Autodesk Inventor part; units mm, degrees
ref_plane "Start Plane" through (0, 0, -13.5858) normal (0, 0, 1) x (1, 0, 0)
ref_plane "End Plane" through (0, 0, 2013.5858) normal (0, 0, 1) x (1, 0, 0)
ref_plane "Work Plane4" through (0, -15.7071, 2014.2929) normal (0, 0.7071, 0.7071) x (1, 0, 0)
ref_plane "Start Plane" through (0, 0, -13.5858) normal (0, 0, 1) x (1, 0, 0)
ref_plane "End Plane" through (0, 0, 2013.5858) normal (0, 0, 1) x (1, 0, 0)
sketch "Sketch" plane through (0, 0, 0) normal (0, 0, 1) x (1, 0, 0)
  line L0 (-15, -12) -> (-15, 12)
  line L1 (-12, 15) -> (12, 15)
  line L2 (15, 12) -> (15, -12)
  line L3 (12, -15) -> (-12, -15)
  arc A0 (-15, -12) -> (-12, -15) centre (-12, -12) ccw
  arc A1 (-12, 15) -> (-15, 12) centre (-12, 12) ccw
  arc A2 (15, 12) -> (12, 15) centre (12, 12) ccw
  arc A3 (12, -15) -> (15, -12) centre (12, -12) ccw
  arc A4 (-12, 13) -> (-13, 12) centre (-12, 12) ccw
  line L4 (-12, 13) -> (12, 13)
  arc A5 (13, 12) -> (12, 13) centre (12, 12) ccw
  line L5 (13, 12) -> (13, -12)
  arc A6 (12, -13) -> (13, -12) centre (12, -12) ccw
  line L6 (12, -13) -> (-12, -13)
  arc A7 (-13, -12) -> (-12, -13) centre (-12, -12) ccw
  line L7 (-13, -12) -> (-13, 12)
  line L8 (0, 21.8698) -> (0, -21.8698) construction
  line L9 (-21.8698, 0) -> (21.8698, 0) construction
  dimension "d7" = 3
  dimension "d10" = 30
  dimension "d11" = 30
  dimension "d12" = 2
  dimension "d15" = 15
  dimension "d16" = 15
extrude "Body" add sketch "Sketch" along normal up to surface (2027.1716 mm away) from surface at -13.5858
sketch "Sketch3" plane through (0, 0, 0) normal (0, 0, 1) x (1, 0, 0)
  line L0 (0, 0) -> (10, 0)
ref_plane "Work Plane3" through (0, 0, 0) normal (0, -1, 0) x (1, 0, 0)
ref_plane "Work Plane4" through (0, -15.7071, 2014.2929) normal (0, 0.7071, 0.7071) x (1, 0, 0)
split "Split1" plane through (0, -15.7071, 2014.2929) removes the side toward (0, 0.7071, 0.7071)
ref_plane "Work Plane5" through (0, -15.7071, -14.2929) normal (0, 0.7071, -0.7071) x (1, 0, 0)
split "Split2" plane through (0, -15.7071, -14.2929) removes the side toward (0, 0.7071, -0.7071)
sketch "Sketch4" plane through (0, 0, 0) normal (0, -1, 0) x (1, 0, 0)
  line L0 (-2, -13.5858) -> (12, -13.5858)
  line L1 (-2, 2013.5858) -> (12, 2013.5858)
  dimension "d18" = 2027.1716
equation "\"d7\" = G_IR"
equation "\"d10\" = G_H"
equation "\"d11\" = G_W"
equation "\"d12\" = G_T"
equation "\"d15\" = 0.5 * d10"
equation "\"d16\" = 0.5 * d11"
equation "\"d3\" = G_L"
equation "\"G_W\" = 30"
equation "\"G_H\" = 30"
equation "\"G_T\" = 2"
equation "\"G_IR\" = 3"
equation "\"G_L\" = d18"
equation "\"G_OFFSET_START\" = 13.58579"
equation "\"G_OFFSET_END\" = 13.58579"
equation "\"d13\" = -G_OFFSET_START"
equation "\"d14\" = G_OFFSET_END + B_L"
properties part number "ISO 12633-2 - 30x30x2 - 2027,17" material "Steel, Mild"
Here's how the part is built. I have some questions about the finished solid (model axes, mm). Coordinates: 2 decimals unless noted, no trailing zeros. Loops run counter-clockwise (first coordinate to the right, second up) from the corner with the lowest first, then second, coordinate; pieces in that order, holes last. Notation, with made-up numbers: (-28.75, -39) -> (-13.75, -39) arc R18 cw to (-13.75, -20) -> close; hole circle Ø3 at (44.5, 77). An arc over 180 degrees is marked (long way). Use one line per item in the form item = value. Start each with the question number.
(1) Will this pin go through, and if not, where does the flat tip stop? pin 1 (10 mm diameter, centred on x = 9, y = -5.5, fed in from -Z).
(2) If we section it at A-A (z = 1587): Please give me the cut outline in (x, y), then the cut area to 3 significant figures.
(3) If we section it at B-B (x = -2.5): Please give me the cut outline in (y, z).
(4) If we section it at C-C (y = -2): Please give me the cut outline in (x, z).
(5) Please list where these lines run through material, in increasing order: line 1 along X through (y, z) = (8, 1045.5); line 2 along Z through (x, y) = (-3.25, -13.5).
Verdict:
q1.pin_1 = -7.09
q2.outline = (-15, -12) arc R3 ccw to (-12, -15) -> (12, -15) arc R3 ccw to (15, -12) -> (15, 12) arc R3 ccw to (12, 15) -> (-12, 15) arc R3 ccw to (-15, 12) -> close; hole (-13, -12) arc R1 ccw to (-12, -13) -> (12, -13) arc R1 ccw to (13, -12) -> (13, 12) arc R1 ccw to (12, 13) -> (-12, 13) arc R1 ccw to (-13, 12) -> close
q2.area = 217 mm²
q3.outline = (-15, -13.59) -> (-13, -11.59) -> (-13, 2011.59) -> (-15, 2013.59) -> close; (13, 14.41) -> (15, 16.41) -> (15, 1983.59) -> (13, 1985.59) -> close
q4.outline = (-15, -0.59) -> (-13, -0.59) -> (-13, 2000.59) -> (-15, 2000.59) -> close; (13, -0.59) -> (15, -0.59) -> (15, 2000.59) -> (13, 2000.59) -> close
q5.line_1 = -15 to -13, 13 to 15
q5.line_2 = -12.09 to 2012.09
